Work out the finished part from the listing and answer in its coordinate system (mm). Coordinates: 2 decimals unless noted, no trailing zeros. Order: outer loops, then holes, each group sorted by start corner. A loop starts at its lowest first (then second) coordinate and runs counter-clockwise, first axis right, second up. Notation, with made-up numbers: M -36,37 L -15,37 A23 cw -15,48 Z; hole C 82,9.25 d8. An arc over 180 degrees is marked long. Write item = value, one per line. Start each with the question number.
Q1. Find section A-A on z = -4.5. Give the vertices of the cut face in (x, y), and give its area (3 significant figures).
Q2. Find section C-C on y = 219. Give the vertices of the cut face in (x, z).
Q3. Straight lines are drawn through the part: line 1 along X through (y, z) = (109, -6.5); line 2 along Y through (x, z) = (59, -4.75); line 3 along X through (y, z) = (96.5, -8.25). For each, find the intervals that lie inside material, in ascending order.
Q4. Each of these flat-tipped pins is pushed along its axis until it touches: P1, Ø4, axis at y = 59.5, z = -9, coming from the +X side; P2, Ø1, axis at y = 82, z = -8, coming from the +X side. Where does it stop, or does it pass through?
Q5. Find section B-B on x = 45. Give the vertices of the cut face in (y, z), and give its area (3 significant figures).
```python
from build123d import *

# Parameters (mm, degrees)
PAD013_DEPTH = 10


with BuildPart() as part:
    # Sketch013 → Pad013 (new body)
    with BuildSketch(Plane.XY):
        Polygon((40.648041, 7.960721), (-60.654729, 67.690055), (-163.033235, 9.82395), (-164.108971, -107.771489), (-62.806201, -167.500823), (39.572305, -109.634718), align=None)
    extrude(amount=-PAD013_DEPTH)


with BuildPart() as part_1:
    # Body013 placement: moved
    add(part.part.moved(Location((164.108971, 167.500823, 0))))


solid = part_1.part
```
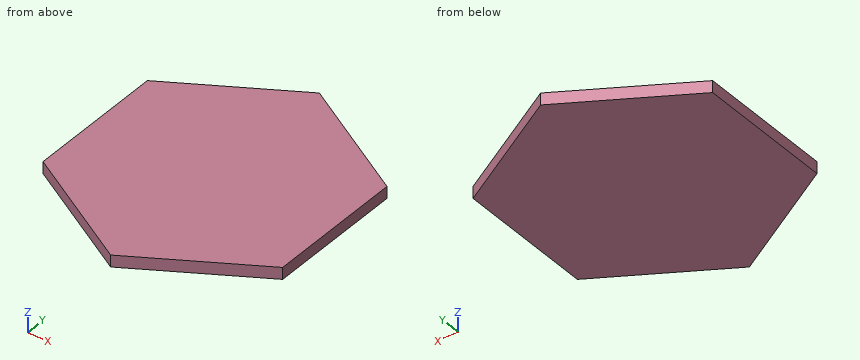
Findings below:
q1.outline = M 0,59.73 L 101.3,0 L 203.68,57.87 L 204.76,175.46 L 103.45,235.19 L 1.08,177.32 Z
q1.area = 35,900 mm^2
q2.outline = M 74.81,-10 L 130.91,-10 L 130.91,0 L 74.81,0 Z
q3.line_1 = 0.45 to 204.15
q3.line_2 = 24.94 to 210.06
q3.line_3 = 0.34 to 204.03
q4.P1 = 203.71
q4.P2 = 203.91
q5.outline = M 33.2,-10 L 202.15,-10 L 202.15,0 L 33.2,0 Z
q5.area = 1,690 mm^2
